Input: part model. Units: mm. Frame: model coordinates. Round coordinates to 2 decimals unless told otherwise and drop trailing zeros. Order: outer loops, then holes, each group sorted by start corner. A loop starts at its lowest first (then second) coordinate and runs counter-clockwise, first axis right, second up.
Item 1: Line query: L1, parallel to Y at x = -42, z = 1.5; L2, parallel to Y at x = -42.5, z = 7; L3, parallel to X at y = 41, z = 6.75. Output: solid intervals per line, ascending.
Item 2: Cut plane A-A on y = -3.5. Output: boundary loops of the cut face in (x, z), then the cut area to 3 significant figures.
Item 3: Cut plane B-B on x = -8. Output: boundary loops of the cut face in (y, z), then the cut area to 3 significant figures.
Item 4: First-contact query: pin 1 (1 mm diameter, centred on x = 36.5, y = -8.5, fed in from -Z); pin 2 (1.5 mm diameter, centred on y = 15, z = 7.5, fed in from +X); pin 3 (1.5 mm diameter, centred on y = -13.5, z = 3, fed in from -X); pin 4 (5 mm diameter, centred on y = -23, z = 8, fed in from -X). Flat tips, straight axial feed; report the tip coordinate or a pass-through.
Item 5: Cut plane C-C on y = 44. Output: boundary loops of the cut face in (x, z).
```python
from build123d import *

# Parameters (mm, degrees)
F1_DEPTH = 10


with BuildPart() as f1:
    # F0 (on Top) → F1 (new body)
    with BuildSketch(Plane.XY):
        with BuildLine():
            ThreePointArc((-64.676278, 0), (-53.560022, 10.275162), (-38.86285, 6.649806))
            ThreePointArc((-38.86285, 6.649806), (-39.244215, 3.79902), (-39.416745, 0.928018))
            ThreePointArc((-39.416745, 0.928018), (-55.864178, -15.231576), (-52.324208, -38.015762))
            ThreePointArc((-52.324208, -38.015762), (-49.370557, -23.16901), (-35.349364, -17.463204))
            ThreePointArc((-35.349364, -17.463204), (-33.982245, -19.993699), (-32.434292, -22.417799))
            ThreePointArc((-32.434292, -22.417799), (-36.242173, -45.158744), (-19.986069, -61.510795))
            ThreePointArc((-19.986069, -61.510795), (-26.323217, -47.763408), (-18.333622, -34.905863))
            ThreePointArc((-18.333622, -34.905863), (-15.740212, -36.149505), (-13.063042, -37.200779))
            ThreePointArc((-13.063042, -37.200779), (-2.776891, -57.836806), (19.986069, -61.510795))
            ThreePointArc((19.986069, -61.510795), (6.778697, -54.113808), (5.68494, -39.015669))
            ThreePointArc((5.68494, -39.015669), (8.514047, -38.497429), (11.297846, -37.774325))
            ThreePointArc((11.297846, -37.774325), (31.74907, -48.423174), (52.324208, -38.015762))
            ThreePointArc((52.324208, -38.015762), (37.291379, -39.794572), (27.532048, -28.222816))
            ThreePointArc((27.532048, -28.222816), (29.516229, -26.140643), (31.343341, -23.919364))
            ThreePointArc((31.343341, -23.919364), (54.147965, -20.513536), (64.676278, 0))
            ThreePointArc((64.676278, 0), (53.560022, -10.275162), (38.86285, -6.649806))
            ThreePointArc((38.86285, -6.649806), (39.244215, -3.79902), (39.416745, -0.928018))
            ThreePointArc((39.416745, -0.928018), (55.864178, 15.231576), (52.324208, 38.015762))
            ThreePointArc((52.324208, 38.015762), (49.370557, 23.16901), (35.349364, 17.463204))
            ThreePointArc((35.349364, 17.463204), (33.982245, 19.993699), (32.434292, 22.417799))
            ThreePointArc((32.434292, 22.417799), (36.242173, 45.158744), (19.986069, 61.510795))
            ThreePointArc((19.986069, 61.510795), (26.323217, 47.763408), (18.333622, 34.905863))
            ThreePointArc((18.333622, 34.905863), (15.740212, 36.149505), (13.063042, 37.200779))
            ThreePointArc((13.063042, 37.200779), (2.776891, 57.836806), (-19.986069, 61.510795))
            ThreePointArc((-19.986069, 61.510795), (-6.778697, 54.113808), (-5.68494, 39.015669))
            ThreePointArc((-5.68494, 39.015669), (-8.514047, 38.497429), (-11.297846, 37.774325))
            ThreePointArc((-11.297846, 37.774325), (-31.74907, 48.423174), (-52.324208, 38.015762))
            ThreePointArc((-52.324208, 38.015762), (-37.291379, 39.794572), (-27.532048, 28.222816))
            ThreePointArc((-27.532048, 28.222816), (-29.516229, 26.140643), (-31.343341, 23.919364))
            ThreePointArc((-31.343341, 23.919364), (-54.147965, 20.513536), (-64.676278, 0))
        make_face()
    extrude(amount=F1_DEPTH)


solid = f1.part
```
From the geometry:
1. L1: y = -18.15 to -0.04, 8.87 to 25.12, 40.87 to 46.31
1. L2: y = -18.33 to -0.26, 9.13 to 25.06, 40.9 to 46.09
1. L3: x = -49.78 to -14.02, -4.95 to 12.82, 24.34 to 37.19
2. outline: (-47.72, 0) - (39.27, 0) - (39.27, 10) - (-47.72, 10) - close; (62.97, 0) - (64.43, 0) - (64.43, 10) - (62.97, 10) - close
2. area: 885 mm2
3. outline: (-52.67, 0) - (38.61, 0) - (38.61, 10) - (-52.67, 10) - close; (55.78, 0) - (62.4, 0) - (62.4, 10) - (55.78, 10) - close
3. area: 979 mm2
4. pin 1: stops at z = 0
4. pin 2: stops at x = 56.03
4. pin 3: stops at x = -55.52
4. pin 4: stops at x = -57.15
5. outline: (-46.17, 0) - (-17.62, 0) - (-17.62, 10) - (-46.17, 10) - close; (-4.36, 0) - (12.21, 0) - (12.21, 10) - (-4.36, 10) - close; (25.63, 0) - (36.58, 0) - (36.58, 10) - (25.63, 10) - close
